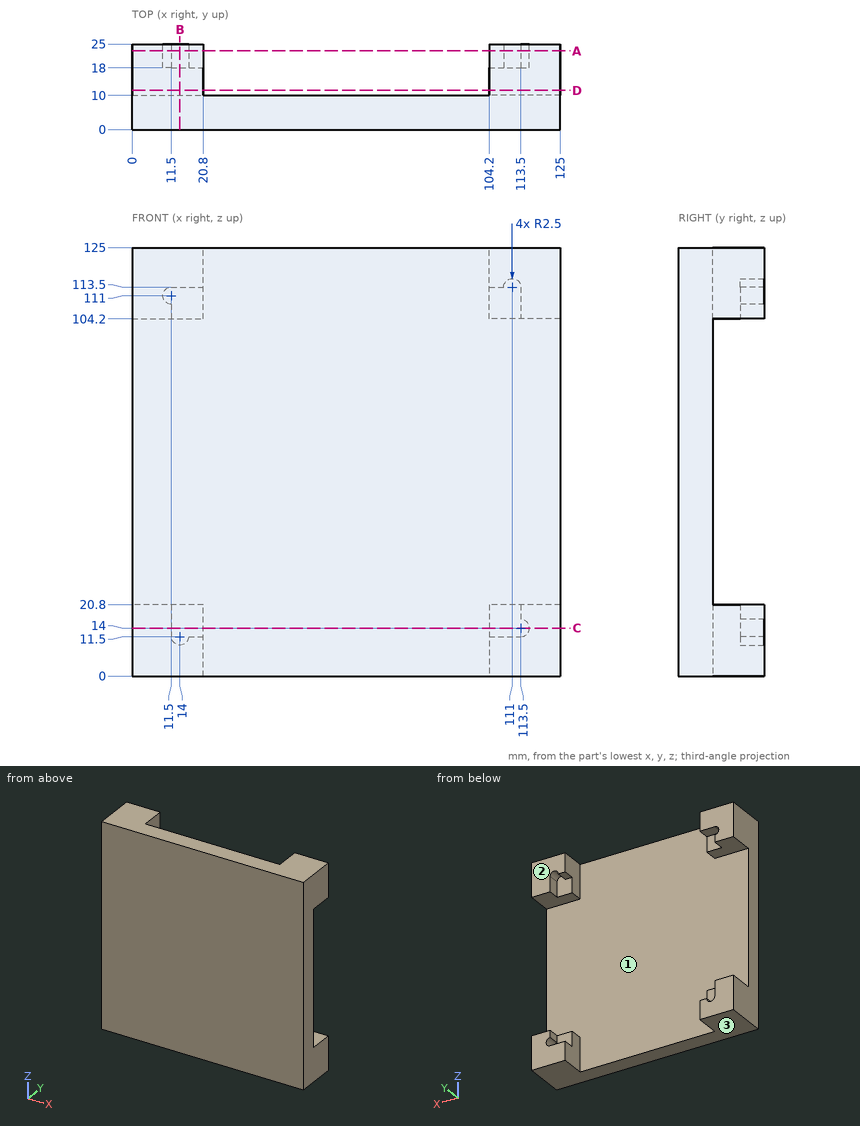
Part print with two shaded views. Sizes in mm from the minimum x, y, z corner. Give positions to 0.01 mm unless a question says otherwise; leave off trailing zeros. Order: outer loops, then holes, each group sorted by start corner. A loop starts at its lowest first (then second) coordinate and runs counter-clockwise, first axis right, second up.
(1) Drill centre lines: L1, parallel to Z at x = 119, y = 16.5; L2, parallel to Z at x = 18, y = 23.5; L3, parallel to Y at x = 12.5, z = 80.5. Where is each one in solid material? Low to high.
(2) Flat gauge pins, fed straight in: pin 1 (6 mm diameter, centred on x = 66.5, y = 15.5, fed in from -Z); pin 2 (10 mm diameter, centred on x = 32.5, z = 105, fed in from +Y); pin 3 (4.5 mm diameter, centred on x = 111, z = 14.5, fed in from +Y). Where does each tip first touch, or does it go through?
(3) Saw through at B-B, the plane x = 14. Give the cut face in (y, z), then the cut area to 3 significant figures.
(4) Saw through at C-C, the plane z = 14. Give the cut face in (x, y), then the cut area to 3 significant figures.
(5) Saw through at A-A, the plane y = 23. Give the cut face in (x, z), then the cut area to 3 significant figures.
(6) Saw through at D-D, the plane y = 11.5. Give the cut face in (x, z).
(7) Mould opens along Z. For the marked faces 1, 2 and 3 say: released by +Z, released by -Z, zero draft, split by the parting line, or undercut.
Results found:
1. L1: z = 0 to 20.8, 104.2 to 125
1. L2: z = 0 to 11.5, 113.5 to 125
1. L3: y = 0 to 10
2. pin 1: passes through
2. pin 2: stops at y = 10
2. pin 3: stops at y = 18
3. outline: (0, 0) - (25, 0) - (25, 9) - (18, 9) - (18, 20.8) - (10, 20.8) - (10, 104.2) - (18, 104.2) - (18, 113.5) - (25, 113.5) - (25, 125) - (0, 125) - close
3. area: 1,730 mm2
4. outline: (0, 0) - (125, 0) - (125, 25) - (116, 25) - (116, 18) - (104.2, 18) - (104.2, 10) - (20.8, 10) - (20.8, 18) - (11.5, 18) - (11.5, 25) - (0, 25) - close
4. area: 1,730 mm2
5. outline: (0, 0) - (20.8, 0) - (20.8, 11.5) - (16.5, 11.5) arc R2.5 cw to (11.5, 11.5) - (11.5, 20.8) - (0, 20.8) - close; (0, 104.2) - (11.5, 104.2) - (11.5, 108.5) arc R2.5 cw to (11.5, 113.5) - (20.8, 113.5) - (20.8, 125) - (0, 125) - close; (104.2, 0) - (125, 0) - (125, 20.8) - (113.5, 20.8) - (113.5, 16.5) arc R2.5 cw to (113.5, 11.5) - (104.2, 11.5) - close; (104.2, 113.5) - (108.5, 113.5) arc R2.5 cw to (113.5, 113.5) - (113.5, 104.2) - (125, 104.2) - (125, 125) - (104.2, 125) - close
5. area: 1,350 mm2
6. outline: (0, 0) - (20.8, 0) - (20.8, 20.8) - (0, 20.8) - close; (0, 104.2) - (20.8, 104.2) - (20.8, 125) - (0, 125) - close; (104.2, 0) - (125, 0) - (125, 20.8) - (104.2, 20.8) - close; (104.2, 104.2) - (125, 104.2) - (125, 125) - (104.2, 125) - close
7. face 1: undercut
7. face 2: zero draft
7. face 3: released by -Z
